from build123d import *

# Parameters (mm, degrees)
CROQUIS1_R                 = 1.5
SALIENTE_EXTRUIR1_DEPTH    = 3
S_LIDO_MOVER_COPIAR1_ANGLE = 90


with BuildPart() as part:
    # Croquis1 → Saliente-Extruir1 (new body)
    with BuildSketch(Plane.XY):
        with BuildLine():
            Line((41421.305272486, -442.43949549), (41421.305272486, -439.43949549))
            Line((41421.305272486, -439.43949549), (41413.305272486, -439.43949549))
            Line((41413.305272486, -439.43949549), (41413.305272486, -437.43949549))
            Line((41413.305272486, -437.43949549), (41419.305272486, -437.43949549))
            Line((41419.305272486, -437.43949549), (41419.305272486, -436.43949549))
            Line((41419.305272486, -436.43949549), (41424.305272486, -436.43949549))
            Line((41424.305272486, -436.43949549), (41424.305272486, -434.43949549))
            Line((41424.305272486, -434.43949549), (41436.305272486, -434.43949549))
            Line((41436.305272486, -434.43949549), (41436.305272486, -437.43949549))
            Line((41436.305272486, -437.43949549), (41440.305272486, -437.43949549))
            Line((41440.305272486, -437.43949549), (41440.305272486, -439.43949549))
            Line((41440.305272486, -439.43949549), (41436.305272486, -439.43949549))
            Line((41436.305272486, -439.43949549), (41436.305272486, -442.43949549))
            Line((41436.305272486, -442.43949549), (41435.066935525, -442.43949549))
            ThreePointArc((41435.066935525, -442.43949549), (41425.333650257, -446.026206837), (41420.255096284, -455.071074438))
            ThreePointArc((41420.255096284, -455.071074438), (41413.38989409, -457.178212126), (41415.921508638, -450.457947386))
            ThreePointArc((41415.921508638, -450.457947386), (41416.286574465, -450.349956968), (41416.584824278, -450.113351733))
            Line((41416.584824278, -450.113351733), (41422.305272486, -443.43949549))
            ThreePointArc((41422.305272486, -443.43949549), (41422.012379267, -442.732388709), (41421.305272486, -442.43949549))
        make_face()
        with Locations((41416.305272486, -454.43949549)):
            Circle(CROQUIS1_R, mode=Mode.SUBTRACT)
    extrude(amount=SALIENTE_EXTRUIR1_DEPTH)


with BuildPart() as part_1:
    # Sólido-Mover/Copiar1: moved
    add(part.part.rotate(Axis((0, -446.43949549, 1.5), (-1, 0, 0)), S_LIDO_MOVER_COPIAR1_ANGLE))


solid = part_1.part
Geometry check sheet. Reference: the model listing, model coordinates, mm. A direction names the side the tool comes from. Round coordinates to 2 decimals unless told otherwise and drop trailing zeros. Loops run counter-clockwise (first coordinate to the right, second up) from the corner with the lowest first, then second, coordinate; pieces in that order, holes last. Notation, with made-up numbers: (61, -21) - (68, -21) arc R21 ccw to (68, -1) - close; hole circle Ø8 at (23.5, 3.25). An arc over 180 degrees is marked (long way). One line per question, with ' | ' between items. Start each with the question number.
1. Cross-section at D-D on z = -5. Record the cut outline in (x, y).
2. Cross-section at A-A on z = 9.5. Record the cut outline in (x, y).
3. Cross-section at C-C on x = 41420.75. Record the cut outline in (y, z), then the cut area to 3 significant figures.
4. Tool access check on faces 4 (the face through (41413.305, -446, -6)), 5 (the face through (41436, -446, -2.5)), 6 (the face through (41438, -446, -7.5)). Record the directions out of +Z, -Z, +X, -X, +Y, -Y that give a thin tool (end or side, any length) a straight path to the whole face; none if there is none.
5. Depth check by flat-ended pin: pin 1 (1.6 mm diameter, centred on y = -447, z = -9, fed in from -X); pin 2 (0.9 mm diameter, centred on x = 41417.5, y = -446.5, fed in from +Z); pin 3 (0.9 mm diameter, centred on y = -447, z = -3.5, fed in from +X). Enter the tip coordinate at first touch or a pass-through.
6. Scan lines: line 1 (Z direction, x = 41437.5, y = -447.1); line 2 (X direction, y = -446.7, z = 9.5); line 3 (X direction, y = -447.25, z = -5). Record each from-to range of solid material in increasing order. Write a range as [from, to].
7. Cross-section at B-B on y = -447.3. Record the cut outline in (x, z), then the cut area to 3 significant figures.
8. Draft check along Z on faces 1 (the face through (41438, -446, -5.5)), 2 (the face through (41421.305, -446, -4)), 3 (the face through (41436.305, -446, -9)). Enter one of: released by +Z, released by -Z, zero draft, split by the parting line, or undercut.
Taken from the geometry:
1) outline: (41421.31, -447.94) - (41436.31, -447.94) - (41436.31, -444.94) - (41421.31, -444.94) - close
2) outline: (41412.31, -447.94) - (41414.81, -447.94) - (41414.81, -444.94) - (41412.31, -444.94) - close; (41417.81, -447.94) - (41420.37, -447.94) - (41420.37, -444.94) - (41417.81, -444.94) - close
3) outline: (-447.94, -8.5) - (-444.94, -8.5) - (-444.94, -5.5) - (-447.94, -5.5) - close; (-447.94, 0.31) - (-444.94, 0.31) - (-444.94, 8.03) - (-447.94, 8.03) - close | area: 32.1 mm²
4) face 4: -Z, -X, +Y, -Y | face 5: +Z, +X, +Y, -Y | face 6: -Z, +X, +Y, -Y
5) pin 1: x = 41419.31 | pin 2: z = 13.43 | pin 3: x = 41436.31
6) line 1: [-7.5, -5.5] | line 2: [41412.31, 41414.81], [41417.81, 41420.37] | line 3: [41421.31, 41436.31]
7) outline: (41413.31, -7.5) - (41419.31, -7.5) - (41419.31, -8.5) - (41424.31, -8.5) - (41424.31, -10.5) - (41436.31, -10.5) - (41436.31, -7.5) - (41440.31, -7.5) - (41440.31, -5.5) - (41436.31, -5.5) - (41436.31, -2.5) - (41435.07, -2.5) arc R15 cw to (41420.26, 10.13) arc R4 ccw (long way) to (41415.92, 5.52) arc R1 cw to (41416.58, 5.17) - (41422.31, -1.5) arc R1 cw to (41421.31, -2.5) - (41421.31, -5.5) - (41413.31, -5.5) - close; hole circle Ø3 at (41416.31, 9.5) | area: 237 mm²
8) face 1: released by +Z | face 2: undercut | face 3: zero draft
